Can you work these out from the model? Positions are in its coordinate system, mm. A direction names the side the tool comes from. Round coordinates to 2 decimals unless told otherwise and drop trailing zeros. Loops run counter-clockwise (first coordinate to the right, second up) from the corner with the lowest first, then second, coordinate; pieces in that order, holes last. Notation, with made-up numbers: (27.5, -22) -> (58.5, -22) arc R34 ccw to (58.5, 13) -> close; hole circle Ø8 at (1, -21.5). An arc over 180 degrees is marked (long way). Answer as a JSON object with one key per item and string values.
Autodesk Inventor part; units mm, degrees
ref_plane "YZ Plane" through (0, 0, 0) normal (1, 0, 0) x (0, 1, 0)
ref_plane "XZ Plane" through (0, 0, 0) normal (0, 1, 0) x (-1, 0, 0)
ref_plane "XY Plane" through (0, 0, 0) normal (0, 0, 1) x (1, 0, 0)
sketch "Sketch5" plane through (0, 0, 0) normal (0, 0, 1) x (1, 0, 0)
  line L0 (52.8, -15.6) -> (52.8, -10.6)
  line L1 (52.8, -10.6) -> (49.8, -10.6)
  line L2 (49.8, -10.6) -> (49.8, -12.6)
  line L3 (44, -12.6) -> (44, -3)
  line L4 (49.8, -3) -> (49.8, -5)
  line L5 (49.8, -5) -> (52.8, -5)
  line L6 (52.8, -5) -> (52.8, 0)
  line L7 (52.8, 0) -> (7.8, 0)
  line L8 (44, -3) -> (49.8, -3)
  line L9 (44, -12.6) -> (49.8, -12.6)
  line L10 (52.8, -15.6) -> (7.8, -15.6)
  line L11 (7.8, -15.6) -> (0, -15.6)
  line L12 (0, -15.6) -> (0, 0)
  line L13 (0, 0) -> (7.8, 0)
  point P0 (7.8, 0)
  dimension "d41" = 5.8
  dimension "d48" = 44
  dimension "d50" = 3
  dimension "d63" = 45
  dimension "d71" = 0
  dimension "d87" = 5.6
  dimension "d88" = 9.6
  dimension "d97" = 15.6
extrude "Extrusion2" add sketch "Sketch5" along normal blind 12
sketch "Sketch8" plane through (0, 0, 0) normal (0, 0, -1) x (-1, 0, 0)
  line L0 (-7.4952, 0) -> (-8.8633, -3.7588)
  line L1 (0, -6.9847) -> (-8.8633, -3.7588)
  line L2 (0, 0) -> (0, -6.9847)
  line L3 (-44, -12.6) -> (-44, -3)
  line L4 (-52.8, 0) -> (0, 0)
  line L5 (-52.8, 0) -> (0, 0)
  line L6 (0, 0) -> (-7.4952, 0)
  dimension "d95" = 4
  dimension "d99" = 35.1367
  dimension "d100" = 110
extrude "Extrusion5" cut sketch "Sketch8" against normal through all
fillet "Fillet2" radius 23 1 edges at (0, -15.6, 6)
equation "\"l1\" = 8"
properties part number "Finray_test_8_Kerbe_10deg"
Q1. I want a section at D-D, the plane y = -1.75. Write out the boundary of the cut face in (x, z), then the cut area to 3 significant figures.
Determined:
{"outline": "(8.13, 0) -> (52.8, 0) -> (52.8, 12) -> (8.13, 12) -> close", "area": "536 mm²"}
Q2. I want a section at C-C, the plane z = 6. Write out the boundary of the cut face in (x, y), then the cut area to 3 significant figures.
Determined:
{"outline": "(0, -6.98) arc R23 ccw to (17.95, -15.6) -> (52.8, -15.6) -> (52.8, -10.6) -> (49.8, -10.6) -> (49.8, -12.6) -> (44, -12.6) -> (44, -3) -> (49.8, -3) -> (49.8, -5) -> (52.8, -5) -> (52.8, 0) -> (7.5, 0) -> (8.86, -3.76) -> close", "area": "659 mm²"}
Q3. I'm going to push flat-ended pins straight in: pin 1 (1 mm diameter, centred on y = -11.5, z = 6, fed in from -X); pin 2 (3 mm diameter, centred on y = -8.5, z = 8, fed in from +X); pin 3 (1 mm diameter, centred on y = -2, z = 7, fed in from -X). Where does each tip first touch, or does it pass through?
Determined:
{"pin 1": "x = 4.15", "pin 2": "x = 44", "pin 3": "x = 8.04"}
Q4. If I drill on L1, parallel to Y at x = 49.5, z = 10; L2, parallel to X at y = -11.5, z = 4.75; L3, parallel to X at y = -8.75, z = 11, over which ranges is the centre line in solid material (lowest first)? Write a range as [from, to].
Determined:
{"L1": "[-15.6, -12.6], [-3, 0]", "L2": "[4.84, 44], [49.8, 52.8]", "L3": "[1.57, 44]"}
Q5. I want a section at A-A, the plane x = 44.5. Write out the boundary of the cut face in (y, z).
Determined:
{"outline": "(-15.6, 0) -> (-12.6, 0) -> (-12.6, 12) -> (-15.6, 12) -> close; (-3, 0) -> (0, 0) -> (0, 12) -> (-3, 12) -> close"}
Q6. I want a section at B-B, the plane y = -11.25. Write out the boundary of the cut face in (x, z), then the cut area to 3 significant figures.
Determined:
{"outline": "(4.49, 0) -> (44, 0) -> (44, 12) -> (4.49, 12) -> close; (49.8, 0) -> (52.8, 0) -> (52.8, 12) -> (49.8, 12) -> close", "area": "510 mm²"}
Q7. On a 3-axis mill with a long thin cutter (end or side, diameter ignored), from which of +Z, -Z, +X, -X, +Y, -Y can I reach the whole of each face in a straight line? I mean faces 1 (the flat face through (8.17, -1.85, 5.92)), 2 (the flat face through (49.8, -4, 6)), 3 (the flat face through (51, -5, 6)). Say none if no direction works.
Determined:
{"face 1": "+Z, -Z, -X", "face 2": "+Z, -Z", "face 3": "+Z, -Z, +X"}
Q8. We'd pull the mould along Y, two halves only. Please class faces 4 (the flat face through (49.8, -12, 6)), 5 (the flat face through (36, -15.6, 6)), 6 (the flat face through (52.8, -3, 6)): pulls with the +Y half, pulls with the -Y half, needs draft (parallel to the pull), parting line crosses it, or undercut.
Determined:
{"face 4": "undercut", "face 5": "pulls with the -Y half", "face 6": "needs draft"}
